Geometry: see drawing. Coordinates: mm, zero at the bounding-box minimum. Coordinates: 2 decimals unless noted, no trailing zeros. Loops run counter-clockwise (first coordinate to the right, second up) from the corner with the lowest first, then second, coordinate; pieces in that order, holes last. Notation, with made-up numbers: (40, -14.5) - (82, -14.5) arc R5 cw to (82, -8.5) - close; hole circle Ø8 at (66.25, 24). An arc over 180 degrees is marked (long way). Use one line per item in the form item = value.
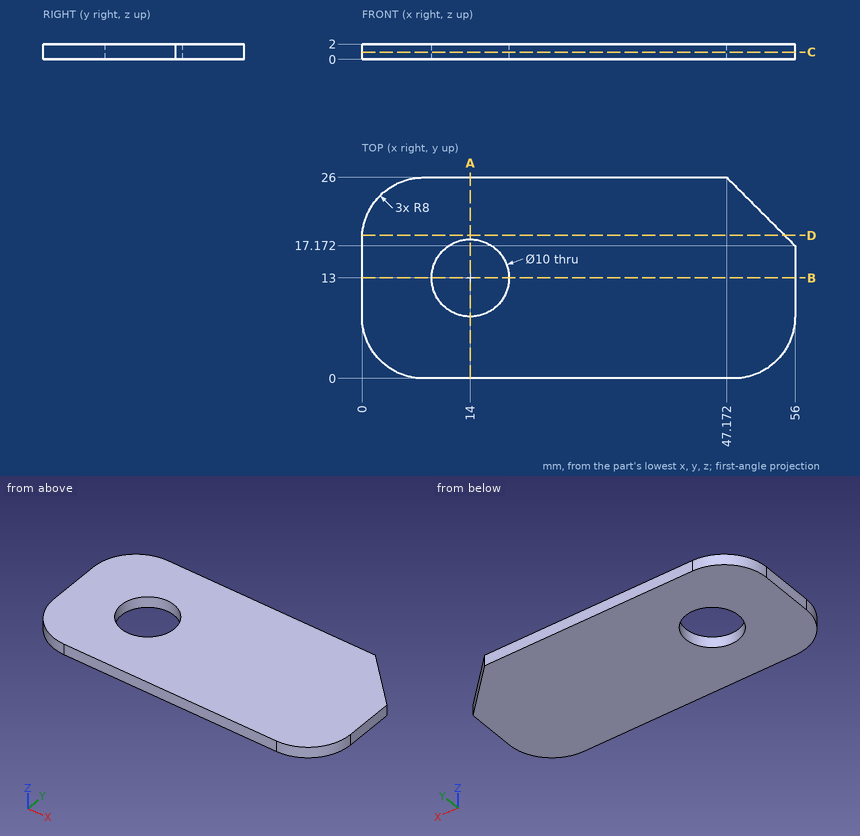
Q1. Cut plane A-A, the plane x = 14. Return loops of the section in (y, z), then the cut area to 3 significant figures.
Check values:
outline = (0, 0) - (8, 0) - (8, 2) - (0, 2) - close; (18, 0) - (26, 0) - (26, 2) - (18, 2) - close
area = 32.0 mm²
Q2. Cut plane C-C, the plane z = 0.95. Return loops of the section in (x, y), then the cut area to 3 significant figures.
Check values:
outline = (0, 8) arc R8 ccw to (8, 0) - (48, 0) arc R8 ccw to (56, 8) - (56, 17.17) - (47.17, 26) - (8, 26) arc R8 ccw to (0, 18) - close; hole circle Ø10 at (14, 13)
area = 1,300 mm²
Q3. Cut plane B-B, the plane y = 13. Return loops of the section in (x, z).
Check values:
outline = (0, 0) - (9, 0) - (9, 2) - (0, 2) - close; (19, 0) - (56, 0) - (56, 2) - (19, 2) - close
Q4. Ray query, line 1 along Y through (x, z) = (14, 0.75); line 2 along X through (y, z) = (9, 1.3); line 3 along Y through (x, z) = (18.5, 1.8) (1 decimal). Return the intervals inside material, ascending. Write a range as [from, to].
Check values:
line_1 = [0, 8], [18, 26]
line_2 = [0, 11], [17, 56]
line_3 = [0, 10.8], [15.2, 26]
Q5. Cut plane D-D, the plane y = 18.5. Return loops of the section in (x, z) (1 decimal).
Check values:
outline = (0, 0) - (54.7, 0) - (54.7, 2) - (0, 2) - close
